```python
from build123d import *

# Parameters (mm, degrees)
CROQUIS1_R              = 70
CROQUIS1_R_2            = 4.5
SALIENTE_EXTRUIR1_DEPTH = 3


with BuildPart() as part:
    # Croquis1 → Saliente-Extruir1 (new body)
    with BuildSketch(Plane(origin=(0, 0, 0), x_dir=(1, 0, 0), z_dir=(0, 1, 0))):
        with Locations(Location((0, 0, 0), (0, 0, 270))):
            Circle(CROQUIS1_R)
        with Locations(Location((0, 0, 0), (0, 0, 270))):
            Circle(CROQUIS1_R_2, mode=Mode.SUBTRACT)
        Polygon((0, 11), (7, 11), (7, 14), (5, 14), (5, 17), (0, 17), (-5, 17), (-5, 14), (-7, 14), (-7, 11), align=None, mode=Mode.SUBTRACT)
        Polygon((24.748737342, 24.748737342), (31.819805153, 17.67766953), (33.941125497, 19.798989873), (19.798989873, 33.941125497), (17.67766953, 31.819805153), align=None, mode=Mode.SUBTRACT)
        Polygon((11, 0), (11, 7), (14, 7), (14, -7), (11, -7), align=None, mode=Mode.SUBTRACT)
        Polygon((-24.748737342, 24.748737342), (-17.67766953, 31.819805153), (-19.798989873, 33.941125497), (-33.941125497, 19.798989873), (-31.819805153, 17.67766953), align=None, mode=Mode.SUBTRACT)
        Polygon((-14, -7), (-11, -7), (-11, 0), (-11, 7), (-14, 7), align=None, mode=Mode.SUBTRACT)
        Polygon((7, -11), (7, -14), (-7, -14), (-7, -11), (0, -11), align=None, mode=Mode.SUBTRACT)
        Polygon((24.748737342, -24.748737342), (17.67766953, -31.819805153), (19.798989873, -33.941125497), (33.941125497, -19.798989873), (31.819805153, -17.67766953), align=None, mode=Mode.SUBTRACT)
        Polygon((-24.748737342, -24.748737342), (-31.819805153, -17.67766953), (-33.941125497, -19.798989873), (-19.798989873, -33.941125497), (-17.67766953, -31.819805153), align=None, mode=Mode.SUBTRACT)
        Polygon((0, 62), (20, 62), (20, 59), (-20, 59), (-20, 62), align=None, mode=Mode.SUBTRACT)
        Polygon((55.861435714, 27.577164466), (27.577164466, 55.861435714), (29.69848481, 57.982756057), (43.840620434, 43.840620434), (57.982756057, 29.69848481), align=None, mode=Mode.SUBTRACT)
        Polygon((59, -20), (59, 20), (62, 20), (62, 0), (62, -20), align=None, mode=Mode.SUBTRACT)
        Polygon((27.577164466, -55.861435714), (55.861435714, -27.577164466), (57.982756057, -29.69848481), (43.840620434, -43.840620434), (29.69848481, -57.982756057), align=None, mode=Mode.SUBTRACT)
        Polygon((-20, -59), (20, -59), (20, -62), (0, -62), (-20, -62), align=None, mode=Mode.SUBTRACT)
        Polygon((-55.861435714, -27.577164466), (-27.577164466, -55.861435714), (-29.69848481, -57.982756057), (-43.840620434, -43.840620434), (-57.982756057, -29.69848481), align=None, mode=Mode.SUBTRACT)
        Polygon((-59, 20), (-59, -20), (-62, -20), (-62, 0), (-62, 20), align=None, mode=Mode.SUBTRACT)
        Polygon((-27.577164466, 55.861435714), (-55.861435714, 27.577164466), (-57.982756057, 29.69848481), (-43.840620434, 43.840620434), (-29.69848481, 57.982756057), align=None, mode=Mode.SUBTRACT)
    extrude(amount=SALIENTE_EXTRUIR1_DEPTH)


solid = part.part
```
For this review, take the finished solid that the model builds, in its own axes (mm). Coordinates: 2 decimals unless noted, no trailing zeros. Loops run counter-clockwise (first coordinate to the right, second up) from the corner with the lowest first, then second, coordinate; pieces in that order, holes last.
1. Add section D-D, the plane z = 23. Give the boundary of the cut face in (x, y), then the cut area to 3 significant figures.
2. For line 1 (X direction, y = 1.1, z = 0); line 2 (X direction, y = 2.15, z = 28.5); line 3 (Z direction, x = -10.5, y = 2.2), list the stretches that pass through material, from the lowest coordinate up.
3. Add section C-C, the plane x = 37. Give the boundary of the cut face in (y, z), then the cut area to 3 significant figures.
4. Mouldability with a two-part tool opening along X and no side actions: class faces 1 (the flat face through (41.52, 1.48, 41.92)), 2 (the flat face through (17, 3, -1)) as +X half, -X half, draft (parallel to the pull), parting line (faces both ways), or undercut.
5. Add section A-A, the plane z = 0. Give the boundary of the cut face in (x, y).
6. Insertion check: P1, Ø0.9, axis at x = 60, y = 1.5, coming from the +Z side; P2, Ø0.6, axis at x = -6.5, y = 1.5, coming from the +Z side; P3, Ø1.5, axis at y = 1, z = 1.5, coming from the +X side; P4, Ø1, axis at x = -13, z = -26.5, coming from the -Y side. Each pin has a flat end and moves straight along its axis. Give the tip position at first contact, or say it passes through.
7. Add section B-B, the plane x = 0. Give the boundary of the cut face in (y, z), then the cut area to 3 significant figures.
Result:
1. outline: (-66.11, 0) - (-30.74, 0) - (-30.74, 3) - (-66.11, 3) - close; (-26.5, 0) - (26.5, 0) - (26.5, 3) - (-26.5, 3) - close; (30.74, 0) - (66.11, 0) - (66.11, 3) - (30.74, 3) - close
1. area: 371 mm2
2. line 1: x = -70 to -62, -59 to -14, -11 to -4.5, 4.5 to 11, 14 to 59, 62 to 70
2. line 2: x = -63.94 to -56.78, -54.94 to -25.24, -21 to 21, 25.24 to 54.94, 56.78 to 63.94
2. line 3: z = -69.21 to -62, -59 to 59, 62 to 69.21
3. outline: (0, -59.42) - (3, -59.42) - (3, -50.68) - (0, -50.68) - close; (0, -46.44) - (3, -46.44) - (3, 46.44) - (0, 46.44) - close; (0, 50.68) - (3, 50.68) - (3, 59.42) - (0, 59.42) - close
3. area: 331 mm2
4. face 1: undercut
4. face 2: draft
5. outline: (-70, 0) - (-62, 0) - (-62, 3) - (-70, 3) - close; (-59, 0) - (-14, 0) - (-14, 3) - (-59, 3) - close; (-11, 0) - (-4.5, 0) - (-4.5, 3) - (-11, 3) - close; (4.5, 0) - (11, 0) - (11, 3) - (4.5, 3) - close; (14, 0) - (59, 0) - (59, 3) - (14, 3) - close; (62, 0) - (70, 0) - (70, 3) - (62, 3) - close
6. P1: stops at z = 36.79
6. P2: stops at z = 69.72
6. P3: stops at x = 70
6. P4: stops at y = 0
7. outline: (0, -70) - (3, -70) - (3, -62) - (0, -62) - close; (0, -59) - (3, -59) - (3, -17) - (0, -17) - close; (0, -11) - (3, -11) - (3, -4.5) - (0, -4.5) - close; (0, 4.5) - (3, 4.5) - (3, 11) - (0, 11) - close; (0, 14) - (3, 14) - (3, 59) - (0, 59) - close; (0, 62) - (3, 62) - (3, 70) - (0, 70) - close
7. area: 348 mm2
